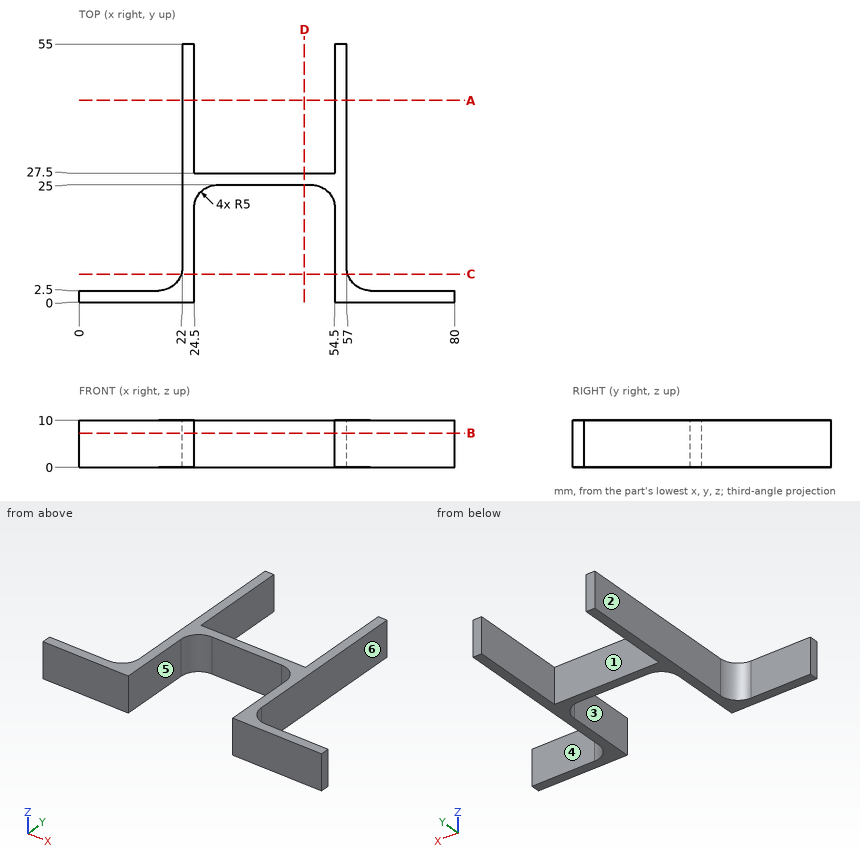
Here's the drawing with two shaded views (mm, measured from the low corner). I have some questions. A direction names the side the tool comes from. Round coordinates to 2 decimals unless told otherwise and drop trailing zeros. Loops run counter-clockwise (first coordinate to the right, second up) from the corner with the lowest first, then second, coordinate; pieces in that order, holes last. Notation, with made-up numbers: (84.25, 40) - (132.25, 40) arc R33 ccw to (132.25, 76) - close; hole circle Ø6 at (-4, -3). An arc over 180 degrees is marked (long way). Use CSV: the item, a comma, the result in double quotes.
Item 1: If we mould it in two halves opening along X, with no side actions, what happens to the marked faces 4, 5 and 6? For each: pulls with the +X half, pulls with the -X half, needs draft (parallel to the pull), parting line crosses it, or undercut.
Here are the results:
face 4,"needs draft"
face 5,"undercut"
face 6,"pulls with the +X half"
Item 2: If we section it at B-B on z = 7.25: List the corners of the cut face in (x, y) for me.
Here are the results:
outline,"(0, 0) - (24.5, 0) - (24.5, 20) arc R5 cw to (29.5, 25) - (49.5, 25) arc R5 cw to (54.5, 20) - (54.5, 0) - (80, 0) - (80, 2.5) - (62, 2.5) arc R5 cw to (57, 7.5) - (57, 55) - (54.5, 55) - (54.5, 27.5) - (24.5, 27.5) - (24.5, 55) - (22, 55) - (22, 7.5) arc R5 cw to (17, 2.5) - (0, 2.5) - close"
Item 3: If we section it at D-D on x = 48: List the corners of the cut face in (y, z) for me.
Here are the results:
outline,"(25, 0) - (27.5, 0) - (27.5, 10) - (25, 10) - close"
Item 4: If we section it at C-C on y = 6: List the corners of the cut face in (x, z) for me, then the cut area to 3 significant figures.
Here are the results:
outline,"(21.77, 0) - (24.5, 0) - (24.5, 10) - (21.77, 10) - close; (54.5, 0) - (57.23, 0) - (57.23, 10) - (54.5, 10) - close"
area,"54.6 mm²"
Item 5: I need wall thicknesses on L1, parallel to X at y = 43, z = 7.5; L2, parallel to Y at x = 73, z = 8; L3, parallel to Y at x = 42.5, z = 8. Which ranges of each line are inside material? Lowest first, please. Write a range as [from, to].
Here are the results:
L1,"x = [22, 24.5], [54.5, 57]"
L2,"y = [0, 2.5]"
L3,"y = [25, 27.5]"
Item 6: If we section it at A-A on y = 43: List the corners of the cut face in (x, z) for me, then the cut area to 3 significant figures.
Here are the results:
outline,"(22, 0) - (24.5, 0) - (24.5, 10) - (22, 10) - close; (54.5, 0) - (57, 0) - (57, 10) - (54.5, 10) - close"
area,"50.0 mm²"
Item 7: Will these pins go through, and if not, where does the flat tip stop? pin 1 (1.5 mm diameter, centred on y = 6, z = 1, fed in from -X); pin 2 (4 mm diameter, centred on y = 16.5, z = 7.5, fed in from -X); pin 3 (3 mm diameter, centred on y = 6.5, z = 5.5, fed in from -X).
Here are the results:
pin 1,"stops at x = 21.47"
pin 2,"stops at x = 22"
pin 3,"stops at x = 21.33"
Item 8: For the marked faces 1, 2 and 3, which set-ups out of +Z, -Z, +X, -X, +Y, -Y let a thin tool reach every point of the face, with its end or its side?
Here are the results:
face 1,"+Z, -Z, +Y"
face 2,"+Z, -Z, -X, +Y"
face 3,"+Z, -Z, -Y"
